Here's how the part is built. I have some questions about the finished solid (model axes, mm). Face numbers are marked on the shaded views. A direction names the side the tool comes from. Give positions to 0.01 mm unless a question says otherwise; leave off trailing zeros. Order: outer loops, then holes, each group sorted by start corner. A loop starts at its lowest first (then second) coordinate and runs counter-clockwise, first axis right, second up. Notation, with made-up numbers: (5.25, 71.25) - (46.25, 71.25) arc R25 ccw to (46.25, 92.25) - close; hole circle Ø1 at (-35.75, 43.5). An arc over 180 degrees is marked (long way). One line per question, with ' | ' between items.
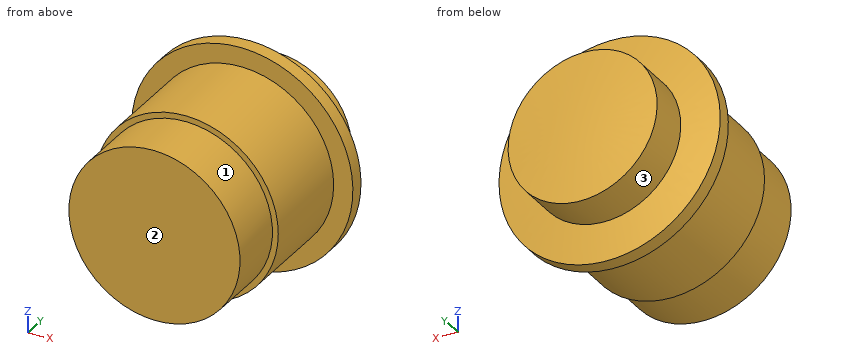
from build123d import *

# Parameters (mm, degrees)
SKETCH1_R           = 7.35
BOSS_EXTRUDE1_DEPTH = 4.8
SKETCH2_R           = 7.85
BOSS_EXTRUDE2_DEPTH = 8.2


with BuildPart() as part:
    # Sketch1 → Boss-Extrude1 (new body)
    with BuildSketch(Plane(origin=(0, 0, 0), x_dir=(1, 0, 0), z_dir=(0, 1, 0))):
        with Locations(Location((0, 0, 0), (0, 0, 270))):
            Circle(SKETCH1_R)
    extrude(amount=BOSS_EXTRUDE1_DEPTH)

    # Sketch2 → Boss-Extrude2 (add)
    with BuildSketch(Plane(origin=(0, 4.8, 0), x_dir=(1, 0, 0), z_dir=(0, 1, 0))):
        with Locations(Location((0, 0, 0), (0, 0, 90))):
            Circle(SKETCH2_R)
    extrude(amount=BOSS_EXTRUDE2_DEPTH)

    # Sketch3 → Revolve2 (revolve)
    with BuildSketch(Plane.XY, mode=Mode.PRIVATE) as revolve2_sk:
        with BuildLine():
            Line((0, 18.610795484), (0, 13))
            Line((0, 13), (-7.85, 13))
            Line((-7.85, 13), (-9.5, 13))
            Line((-9.5, 13), (-9.5, 14.2))
            ThreePointArc((-9.5, 14.2), (-7.953922053, 14.474092821), (-6.4, 14.699503876))
            Line((-6.4, 14.699503876), (-6.4, 18.199503876))
            ThreePointArc((-6.4, 18.199503876), (-3.206601035, 18.507866639), (0, 18.610795484))
        make_face()
    revolve(revolve2_sk.sketch.rotate(Axis((0, 15.200891001, 0), (0, -1, 0)), 270), axis=Axis((0, 15.200891001, 0), (0, -1, 0)))


solid = part.part
1) On a 3-axis mill with a long thin cutter (end or side, diameter ignored), from which of +Z, -Z, +X, -X, +Y, -Y can I reach the whole of each face in a straight line? I mean the marked faces 1, 2 and 3. Say none if no direction works.
Model answer:
face 1: -Y | face 2: +Z, -Z, +X, -X, -Y | face 3: +Y
2) I'm going to push flat-ended pins straight in: P1, Ø1, axis at x = 2.5, z = 2.5, coming from the +Y side; P2, Ø6, axis at y = 8, z = 1.5, coming from the -X side; P3, Ø10, axis at x = 6.5, z = 2.5, coming from the +Y side. Where does each tip first touch, or does it pass through?
Model answer:
P1: stops at y = 18.52 | P2: stops at x = -7.85 | P3: stops at y = 18.57
3) I want a section at C-C (y = 6.75). List the corners of the cut face in (x, z) for me.
Model answer:
outline: circle Ø15.7 at (0, 0)
4) I want a section at D-D (x = 5). List the corners of the cut face in (y, z) for me (1 decimal), plus the area to 3 significant figures.
Model answer:
outline: (0, -5.4) - (4.8, -5.4) - (4.8, -6.1) - (13, -6.1) - (13, -8.1) - (14.2, -8.1) arc R49.7 ccw to (14.7, -4) - (18.2, -4) arc R49.7 ccw to (18.2, 4) - (14.7, 4) arc R49.7 ccw to (14.2, 8.1) - (13, 8.1) - (13, 6.1) - (4.8, 6.1) - (4.8, 5.4) - (0, 5.4) - close | area: 205 mm2
5) Please list where these lines run through material, in increasing order: L1, parallel to Y at x = 7.75, z = -1.5; L2, parallel to Z at x = 4.75, y = 17.75; L3, parallel to Z at x = 0.25, y = 4.75.
Model answer:
L1: y = 13 to 14.48 | L2: z = -4.29 to 4.29 | L3: z = -7.35 to 7.35
6) I want a section at B-B (z = 0). List the corners of the cut face in (x, y) for me, plus the area to 3 significant figures.
Model answer:
outline: (-9.5, 13) - (-7.85, 13) - (-7.85, 4.8) - (-7.35, 4.8) - (-7.35, 0) - (7.35, 0) - (7.35, 4.8) - (7.85, 4.8) - (7.85, 13) - (9.5, 13) - (9.5, 14.2) arc R50 ccw to (6.4, 14.7) - (6.4, 18.2) arc R50 ccw to (-6.4, 18.2) - (-6.4, 14.7) arc R50 ccw to (-9.5, 14.2) - close | area: 278 mm2
7) I want a section at A-A (x = 0). List the corners of the cut face in (y, z) for me, plus the area to 3 significant figures.
Model answer:
outline: (0, -7.35) - (4.8, -7.35) - (4.8, -7.85) - (13, -7.85) - (13, -9.5) - (14.2, -9.5) arc R50 ccw to (14.7, -6.4) - (18.2, -6.4) arc R50 ccw to (18.2, 6.4) - (14.7, 6.4) arc R50 ccw to (14.2, 9.5) - (13, 9.5) - (13, 7.85) - (4.8, 7.85) - (4.8, 7.35) - (0, 7.35) - close | area: 278 mm2
